Part model, mm, in its own coordinate system. A direction names the side the tool comes from. Give positions to 0.01 mm unless a question says otherwise; leave off trailing zeros. Write each loop counter-clockwise with the first axis right and the second up, starting at its lowest first coordinate (ties: lowest second). Pieces come first, ordered by that corner, then holes. Notation, with made-up numbers: M -19.5,56 L 3.5,56 A34 ccw 3.5,90 Z; hole C -12.5,-24 d4. An arc over 180 degrees is marked long. Use CSV: the item, a comma, the result in double quotes. Start each with the question number.
Item 1: Mould opens along Y. For faces 4 (the cylindrical face through (-1.542, -0.143, 15.747)), 5 (the cylindrical face through (-4.3, -0.1, 16.5)), 6 (the cylindrical face through (1.246, 2.681, -6.466)), 7 (the cylindrical face through (-4, -10, 0)) say: released by +Y, released by -Y, zero draft, split by the parting line, or undercut.
Item 2: Drill centre lines: line 1 (Z direction, x = -1, y = 1.75); line 2 (Y direction, x = 0, z = -14); line 3 (Z direction, x = -6.25, y = -3.5). Where is each one in solid material? Low to high. Write a range as [from, to].
Item 3: Cut at D-D (x = -0.5). List the corners of the cut face in (y, z).
Item 4: Cut at C-C (z = 0). List the corners of the cut face in (x, y), then the cut area to 3 significant figures.
Item 5: Which spindle directions (+Z, -Z, +X, -X, +Y, -Y) get a long thin tool onto all of the face, cutting with end or side? Do faces 1 (the flat face through (-4.33, -6.104, -9.677)), 2 (the flat face through (-4.5, 1, 14)), 3 (the cylindrical face through (-4.68, 7.81, -1.73)). Say none if no direction does.
Item 6: Pin check, flat tips, straight feed: pin 1 (3.5 mm diameter, centred on y = 0, z = -12.5, fed in from -X); pin 2 (1 mm diameter, centred on x = -3, z = -10, fed in from -Y); pin 3 (2 mm diameter, centred on x = -3, z = 5, fed in from +Y). Stop position of each tip, or through.
Item 7: Cut at A-A (y = 0). Count the separate pieces of the cut face and the enclosed holes in it, then the cut area to 3 significant figures.
Item 8: Cut at B-B (x = -9). List the corners of the cut face in (y, z).
Autodesk Inventor part; units mm, degrees
ref_plane "Work Plane1" through (-10, 0, 0) normal (1, 0, 0) x (0, 1, 0)
ref_plane "XZ Plane" through (0, 0, 0) normal (0, 1, 0) x (-1, 0, 0)
ref_plane "XY Plane" through (0, 0, 0) normal (0, 0, 1) x (1, 0, 0)
ref_plane "Work Plane1" through (-10, 0, 0) normal (1, 0, 0) x (0, 1, 0)
sketch "Sketch1" plane through (-10, 0, 0) normal (1, 0, 0) x (0, 1, 0)
  line L0 (3.5091, 14.42) -> (8.7727, 4.8)
  arc A0 (-8.7727, 4.8) -> (-8.7727, -4.8) centre (0, 0) ccw
  line L1 (8.7727, -4.8) -> (3.5091, -14.42)
  arc A1 (3.5091, 14.42) -> (-3.5091, 14.42) centre (0, 12.5) ccw
  line L2 (-3.5091, -14.42) -> (-8.7727, -4.8)
  arc A2 (8.7727, -4.8) -> (8.7727, 4.8) centre (0, 0) ccw
  line L3 (-8.7727, 4.8) -> (-3.5091, 14.42)
  arc A3 (-3.5091, -14.42) -> (3.5091, -14.42) centre (0, -12.5) ccw
extrude "Extrusion1" add sketch "Sketch1" along normal blind 11.5
hole "Hole4" at (1.5, 0, 0) direction (-1, 0, 0) diameter 14 depth 11.5
hole "Hole3" at (1.5, 0, -12.5) direction (-1, 0, 0) diameter 3.2 depth 11.5 counterbore diameter 6.5 counterbore depth 6
sketch "Sketch3" plane through (1.5, 0, 0) normal (1, 0, 0) x (0, 0, -1)
  point P0 (12.5, 0)
hole "Hole2" at (1.5, 0, 12.5) direction (-1, 0, 0) diameter 3.2 depth 11.5 counterbore diameter 6.5 counterbore depth 6
sketch "Sketch2" plane through (1.5, 0, 0) normal (1, 0, 0) x (0, 0, -1)
  point P0 (0, 0)
hole "Hole1" at (-10, 0, 0) direction (1, 0, 0) diameter 16 depth 10 tip angle 90
chamfer "Chamfer3" distance 0.5 angle 45 1 edges at (-10, 0, -10.9)
chamfer "Chamfer2" distance 0.5 angle 45 1 edges at (-10, 0, 14.1)
chamfer "Chamfer1" distance 0.5 angle 45 1 edges at (-10, 0, -8)
sketch "Sketch4" plane through (1.5, 0, 0) normal (1, 0, 0) x (0, 0, -1)
  point P0 (-12.5, 0)
sketch "Sketch5" plane through (-10, 0, 0) normal (1, 0, 0) x (0, 1, 0)
  point P0 (0, 0)
properties part number "XY Drive Bearing Holder"
Worked answers:
1,face 4,"undercut"
1,face 5,"split by the parting line"
1,face 6,"undercut"
1,face 7,"released by -Y"
2,line 1,"z = [-16.1, -15.24], [-9.76, -7.81], [7.81, 9.76], [15.24, 16.1]"
2,line 2,"y = [-3.74, -2.88], [2.88, 3.74]"
2,line 3,"z = [-14.44, -7.19], [7.19, 14.44]"
3,outline,"M -8.77,-4.8 L -3.51,-14.42 A4 ccw 3.51,-14.42 L 8.77,-4.8 A10 ccw 8.77,4.8 L 3.51,14.42 A4 ccw -3.51,14.42 L -8.77,4.8 A10 ccw Z; hole C 0,0 d16; hole C 0,-12.5 d6.5; hole C 0,12.5 d6.5"
4,outline,"M -10,-10 L 1.5,-10 L 1.5,-7 L 1,-7 L 0,-8 L -9.5,-8 L -10,-8.5 Z; M -10,8.5 L -9.5,8 L 0,8 L 1,7 L 1.5,7 L 1.5,10 L -10,10 Z"
4,area,"47.8 mm^2"
5,face 1,"-Z, +X, -X, -Y"
5,face 2,"+X"
5,face 3,"-X"
6,pin 1,"stops at x = -9.65"
6,pin 2,"stops at y = -6.2"
6,pin 3,"stops at y = 9.17"
7,separate pieces,"4"
7,enclosed holes,"0"
7,area,"83.6 mm^2"
8,outline,"M -8.77,-4.8 L -3.51,-14.42 A4 ccw 3.51,-14.42 L 8.77,-4.8 A10 ccw 8.77,4.8 L 3.51,14.42 A4 ccw -3.51,14.42 L -8.77,4.8 A10 ccw Z; hole C 0,0 d16; hole C 0,-12.5 d3.2; hole C 0,12.5 d3.2"
